from build123d import *

# Parameters (mm, degrees)
BOSS_EXTRUDE1_DEPTH = 6.35


with BuildPart() as part:
    # Sketch1 → Boss-Extrude1 (new body)
    with BuildSketch(Plane(origin=(0, 0, 0), x_dir=(1, 0, 0), z_dir=(0, 1, 0))):
        with BuildLine():
            ThreePointArc((-109.011585227, 263.177247511), (-55.57362422, 279.387475761), (0, 284.861))
            Line((0, 284.861), (0, 288.036))
            Line((0, 288.036), (6.35, 288.036))
            Line((6.35, 288.036), (6.35, 291.211))
            Line((6.35, 291.211), (0, 291.211))
            Line((0, 291.211), (0, 294.386))
            ThreePointArc((0, 294.386), (-57.431859537, 288.729455557), (-112.65664492, 271.977200058))
            Line((-112.65664492, 271.977200058), (-111.441625022, 269.043882542))
            Line((-111.441625022, 269.043882542), (-109.011585227, 263.177247511))
        make_face()
        with BuildLine():
            ThreePointArc((-269.043882542, 111.441625022), (-205.917272856, 205.917272856), (-111.441625022, 269.043882542))
            Line((-111.441625022, 269.043882542), (-112.65664492, 271.977200058))
            ThreePointArc((-112.65664492, 271.977200058), (-208.162336886, 208.162336886), (-271.977200058, 112.65664492))
            Line((-271.977200058, 112.65664492), (-269.043882542, 111.441625022))
        make_face()
        with BuildLine():
            Line((-263.177247511, 109.011585227), (-269.043882542, 111.441625022))
            Line((-269.043882542, 111.441625022), (-271.977200058, 112.65664492))
            ThreePointArc((-271.977200058, 112.65664492), (-288.729455557, 57.431859537), (-294.386, 0))
            Line((-294.386, 0), (-291.211, 0))
            Line((-291.211, 0), (-291.211, 6.35))
            Line((-291.211, 6.35), (-288.036, 6.35))
            Line((-288.036, 6.35), (-288.036, 0))
            Line((-288.036, 0), (-284.861, 0))
            ThreePointArc((-284.861, 0), (-279.387475761, 55.57362422), (-263.177247511, 109.011585227))
        make_face()
    extrude(amount=BOSS_EXTRUDE1_DEPTH)


solid = part.part
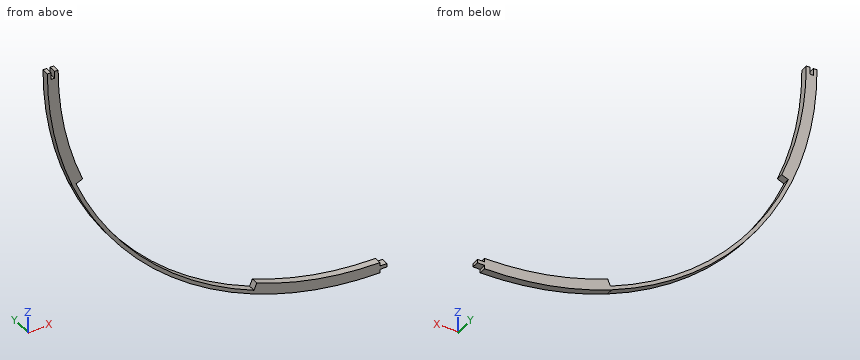
The model under review builds one solid part; all positions refer to its coordinate system, in mm. Give positions to 0.01 mm unless a question says otherwise; leave off trailing zeros. Order: outer loops, then holes, each group sorted by start corner. A loop starts at its lowest first (then second) coordinate and runs counter-clockwise, first axis right, second up. Notation, with made-up numbers: M 56.25,0.5 L 84.25,0.5 A36 cw 84.25,35.5 Z; hole C 4.5,-5.5 d4. An arc over 180 degrees is marked long. Use one line per item in the form item = value. Start each with the question number.
Item 1: We need section A-A on y = 5. Give the boundary of the cut face in (x, z).
Item 2: Insertion check: pin 1 Ø1 at (x, y) = (-208, 4) entering from -Z; pin 2 Ø2.5 at (y, z) = (4.5, -286.5) entering from +X; pin 3 Ø2 at (y, z) = (5.5, -131) entering from +X. Each pin has a flat end and moves straight along its axis. Give the tip position at first contact, or say it passes through.
Item 3: We need section B-B on x = -31. Give the boundary of the cut face in (y, z), plus the area to 3 significant figures.
Item 4: We need section C-C on z = -82.5. Give the boundary of the cut face in (x, y).
Item 5: To check wall thickness, follow line 1 along Z through (x, y) = (-115, 5.25); line 2 along X through (y, z) = (5, -186); line 3 along X through (y, z) = (4.5, -166). State the ranges of each line that lie inside material, in increasing order. Write a range as from..to.
Completed:
q1.outline = M -294.39,0 A294.39 ccw 0,-294.39 L 0,-291.21 L 6.35,-291.21 L 6.35,-288.04 L 0,-288.04 L 0,-284.86 A284.86 cw -109.01,-263.18 L -111.44,-269.04 A291.21 cw -269.04,-111.44 L -263.18,-109.01 A284.86 cw -284.86,0 L -288.04,0 L -288.04,-6.35 L -291.21,-6.35 L -291.21,0 Z
q2.pin_1 = -208.82
q2.pin_2 = 0
q2.pin_3 = -259.58
q3.outline = M 0,-292.75 L 6.35,-292.75 L 6.35,-283.17 L 0,-283.17 Z
q3.area = 60.8 mm²
q4.outline = M -282.59,0 L -272.65,0 L -272.65,6.35 L -282.59,6.35 Z
q5.line_1 = -270.99..-267.54
q5.line_2 = -228.18..-224.07
q5.line_3 = -243.12..-239.27
